Model file for the job. Use its own axes, mm. A direction names the side the tool comes from. Coordinates: 2 decimals unless noted, no trailing zeros. Loops run counter-clockwise (first coordinate to the right, second up) from the corner with the lowest first, then second, coordinate; pieces in that order, holes last. Notation, with made-up numbers: (-40, -40) -> (-30, -40) arc R32 cw to (-30, -8) -> close; hole circle Ø4 at (-7.5, 16). An arc over 180 degrees is marked (long way). Use one line per item in the form item = value.
```python
from build123d import *


with BuildPart() as part:
    # Sketch1 → Revolve1 (revolve)
    with BuildSketch(Plane(origin=(0, 0, 0), x_dir=(0, 0, -1), z_dir=(1, 0, 0)), mode=Mode.PRIVATE) as revolve1_sk:
        Polygon((0, 0), (0, 2), (3, 2), (3, 2.5), (10, 2.5), (10, 3), (73, 3), (73, 2.5), (80, 2.5), (80, 2), (83, 2), (83, 0), align=None)
    revolve(revolve1_sk.sketch.rotate(Axis((0, 0, 10.073341037), (0, 0, -1)), 90), axis=Axis((0, 0, 10.073341037), (0, 0, -1)))


solid = part.part
```
Q1. Wall check: line 1 along Y through (x, z) = (-0.3, -53.5); line 2 along Z through (x, y) = (1.7, 1.4); line 3 along Z through (x, y) = (-2.3, 1.25). Give the ranges that are in metal, low to high.
Result:
line_1 = -2.98 to 2.98
line_2 = -80 to -3
line_3 = -73 to -10
Q2. Band-saw the part on C-C, the plane z = -76.5. Write the cut outline in (x, y).
Result:
outline = circle Ø5 at (0, 0)
Q3. Band-saw the part on D-D, the plane z = -51.5. Write the cut outline in (x, y).
Result:
outline = circle Ø6 at (0, 0)
Q4. Pin check, flat tip, straight feed: pin 1 Ø1 at (y, z) = (-1.5, -58) entering from -X. Stop position of the tip, or through.
Result:
pin_1 = -2.83
Q5. Which spindle directions (+Z, -Z, +X, -X, +Y, -Y) get a long thin tool onto all of the face, cutting with end or side? Do faces 1 (the face through (2.86, -0.9, -41.94)), 2 (the face through (-2.5, -0.1, -6.5)), 3 (the face through (-2, -2, -73)). Say none if no direction does.
Result:
face_1 = +Z, -Z
face_2 = +Z
face_3 = -Z
Q6. Band-saw the part on A-A, the plane x = 0. Write the cut outline in (y, z).
Result:
outline = (-3, -73) -> (-2.5, -73) -> (-2.5, -80) -> (-2, -80) -> (-2, -83) -> (2, -83) -> (2, -80) -> (2.5, -80) -> (2.5, -73) -> (3, -73) -> (3, -10) -> (2.5, -10) -> (2.5, -3) -> (2, -3) -> (2, 0) -> (-2, 0) -> (-2, -3) -> (-2.5, -3) -> (-2.5, -10) -> (-3, -10) -> close
